Can you work these out from the model? Positions are in its coordinate system, mm. A direction names the side the tool comes from. Give positions to 0.01 mm unless a question says otherwise; leave off trailing zeros. Loops run counter-clockwise (first coordinate to the right, second up) from the corner with the lowest first, then second, coordinate; pieces in that order, holes last. Notation, with made-up numbers: (38.25, 26.25) -> (56.25, 26.25) arc R24 cw to (56.25, 45.25) -> close; hole circle Ø3 at (21, -29). An arc over 180 degrees is marked (long way). Return JSON: item names as keys, results as strings. Group by question number.
Q1. Suppose I cut it at B-B, the plane y = 14.5. Please give me the cut outline in (x, z) (3 decimals), and give its area (3 significant figures).
Q2. Suppose I cut it at C-C, the plane x = 44.5. Please give me the cut outline in (y, z).
Q3. I need wall thicknesses on line 1 along X through (y, z) = (14.75, 5.5) (3 decimals); line 2 along Y through (x, z) = (46.5, 6); line 3 along Z through (x, y) = (28, 4.75). Which ranges of each line are inside material? Lowest first, please. Write a range as [from, to].
Q4. Thinking about a two-plate mould opening in X: for faces 1 (the cylindrical face through (0.285, 1.014, 7.699)), 2 (the cylindrical face through (49.324, 14.986, 7.715)), 3 (the flat face through (2, 15, 8)), which applies, pulls with the +X half, pulls with the -X half, needs draft (parallel to the pull), parting line crosses it, or undercut?
Q5. Will these pins go through, and if not, where does the flat tip stop? pin 1 (8 mm diameter, centred on x = 20.5, y = 3.5, fed in from -Z); pin 2 (1.4 mm diameter, centred on x = 51, y = 1.5, fed in from +Z); pin 3 (8 mm diameter, centred on x = 29.5, y = 11.5, fed in from +Z).
Q6. Which directions (+Z, -Z, +X, -X, +Y, -Y) give clear straight access to the entire face, cutting with the end or side of a thin tool? Please do faces 4 (the flat face through (49, 14, 5)), 5 (the flat face through (50, 1, 2)), 6 (the cylindrical face through (55.215, 15.014, 7.699)).
Q7. Suppose I cut it at A-A, the plane z = 3.75. Count the separate pieces of the cut face and the enclosed holes in it, and give its area (3 significant figures).
```python
from build123d import *

# Parameters (mm, degrees)
BOX001_W     = 1.75
BOX001_H     = 2
BOX001_DEPTH = 10
BOX_W        = 10
BOX_H        = 2
BOX_DEPTH    = 8
FILLET_R     = 1
BOX003_W     = 1.75
BOX003_H     = 2
BOX003_DEPTH = 10
BOX002_W     = 10
BOX002_H     = 2
BOX002_DEPTH = 8
FILLET001_R  = 1
BOX005_W     = 1.75
BOX005_H     = 2
BOX005_DEPTH = 10
BOX004_W     = 10
BOX004_H     = 2
BOX004_DEPTH = 8
FILLET002_R  = 1
BOX007_W     = 1.75
BOX007_H     = 2
BOX007_DEPTH = 10
BOX006_W     = 10
BOX006_H     = 2
BOX006_DEPTH = 8
FILLET003_R  = 1
BOX008_W     = 55.5
BOX008_H     = 16
BOX008_DEPTH = 1.75


with BuildPart() as cube001:
    # Box001 → Box001 (new body)
    with BuildSketch(Plane(origin=(4.125, 0, 2), x_dir=(1, 0, 0), z_dir=(0, 0, 1))):
        with Locations((0.875, 1)):
            Rectangle(BOX001_W, BOX001_H)
    extrude(amount=BOX001_DEPTH)


with BuildPart() as post01:
    # Box → Box (new body)
    with BuildSketch(Plane.XY):
        with Locations((5, 1)):
            Rectangle(BOX_W, BOX_H)
    extrude(amount=BOX_DEPTH)

    # Cut: cut Cube001
    add(cube001.part, mode=Mode.SUBTRACT)

    # Fillet
    fillet_edges = [post01.edges().sort_by_distance(p)[0] for p in [
        (0, 1, 8),
        (4.125, 1, 8),
        (10, 1, 8),
        (5.875, 1, 8),
    ]]
    fillet(fillet_edges, radius=FILLET_R)


with BuildPart() as cube003:
    # Box003 → Box003 (new body)
    with BuildSketch(Plane(origin=(4.125, 0, 2), x_dir=(1, 0, 0), z_dir=(0, 0, 1))):
        with Locations((0.875, 1)):
            Rectangle(BOX003_W, BOX003_H)
    extrude(amount=BOX003_DEPTH)


with BuildPart() as post002:
    # Box002 → Box002 (new body)
    with BuildSketch(Plane.XY):
        with Locations((5, 1)):
            Rectangle(BOX002_W, BOX002_H)
    extrude(amount=BOX002_DEPTH)

    # Cut001: cut Cube003
    add(cube003.part, mode=Mode.SUBTRACT)

    # Fillet001
    fillet001_edges = [post002.edges().sort_by_distance(p)[0] for p in [
        (0, 1, 8),
        (4.125, 1, 8),
        (10, 1, 8),
        (5.875, 1, 8),
    ]]
    fillet(fillet001_edges, radius=FILLET001_R)


with BuildPart() as post002_1:
    # Fillet001 placement: moved
    add(post002.part.moved(Location((0, 14, 0))))


with BuildPart() as cube005:
    # Box005 → Box005 (new body)
    with BuildSketch(Plane(origin=(4.125, 0, 2), x_dir=(1, 0, 0), z_dir=(0, 0, 1))):
        with Locations((0.875, 1)):
            Rectangle(BOX005_W, BOX005_H)
    extrude(amount=BOX005_DEPTH)


with BuildPart() as post003:
    # Box004 → Box004 (new body)
    with BuildSketch(Plane.XY):
        with Locations((5, 1)):
            Rectangle(BOX004_W, BOX004_H)
    extrude(amount=BOX004_DEPTH)

    # Cut002: cut Cube005
    add(cube005.part, mode=Mode.SUBTRACT)

    # Fillet002
    fillet002_edges = [post003.edges().sort_by_distance(p)[0] for p in [
        (0, 1, 8),
        (4.125, 1, 8),
        (10, 1, 8),
        (5.875, 1, 8),
    ]]
    fillet(fillet002_edges, radius=FILLET002_R)


with BuildPart() as post003_1:
    # Fillet002 placement: moved
    add(post003.part.moved(Location((45.5, 0, 0))))


with BuildPart() as cube007:
    # Box007 → Box007 (new body)
    with BuildSketch(Plane(origin=(4.125, 0, 2), x_dir=(1, 0, 0), z_dir=(0, 0, 1))):
        with Locations((0.875, 1)):
            Rectangle(BOX007_W, BOX007_H)
    extrude(amount=BOX007_DEPTH)


with BuildPart() as post004:
    # Box006 → Box006 (new body)
    with BuildSketch(Plane.XY):
        with Locations((5, 1)):
            Rectangle(BOX006_W, BOX006_H)
    extrude(amount=BOX006_DEPTH)

    # Cut003: cut Cube007
    add(cube007.part, mode=Mode.SUBTRACT)

    # Fillet003
    fillet003_edges = [post004.edges().sort_by_distance(p)[0] for p in [
        (0, 1, 8),
        (4.125, 1, 8),
        (10, 1, 8),
        (5.875, 1, 8),
    ]]
    fillet(fillet003_edges, radius=FILLET003_R)


with BuildPart() as post004_1:
    # Fillet003 placement: moved
    add(post004.part.moved(Location((45.5, 14, 0))))


with BuildPart() as axlejig:
    # Box008 → Box008 (new body)
    with BuildSketch(Plane.XY):
        with Locations((27.75, 8)):
            Rectangle(BOX008_W, BOX008_H)
    extrude(amount=BOX008_DEPTH)

    # Fusion: union post01, post002, post003, post004
    add(post01.part)
    add(post002_1.part)
    add(post003_1.part)
    add(post004_1.part)


solid = axlejig.part
```
Ans:
{
 "1": {"outline": "(0, 0) -> (55.5, 0) -> (55.5, 7) arc R1 ccw to (54.5, 8) -> (52.375, 8) arc R1 ccw to (51.375, 7) -> (51.375, 2) -> (49.625, 2) -> (49.625, 7) arc R1 ccw to (48.625, 8) -> (46.5, 8) arc R1 ccw to (45.5, 7) -> (45.5, 1.75) -> (10, 1.75) -> (10, 7) arc R1 ccw to (9, 8) -> (6.875, 8) arc R1 ccw to (5.875, 7) -> (5.875, 2) -> (4.125, 2) -> (4.125, 7) arc R1 ccw to (3.125, 8) -> (1, 8) arc R1 ccw to (0, 7) -> close", "area": "199 mm^2"},
 "2": {"outline": "(0, 0) -> (16, 0) -> (16, 1.75) -> (0, 1.75) -> close"},
 "3": {"line 1": "x = [0, 4.125], [5.875, 10], [45.5, 49.625], [51.375, 55.5]", "line 2": "y = [0, 2], [14, 16]", "line 3": "z = [0, 1.75]"},
 "4": {"face 1": "pulls with the -X half", "face 2": "undercut", "face 3": "needs draft"},
 "5": {"pin 1": "stops at z = 0", "pin 2": "stops at z = 7.74", "pin 3": "stops at z = 1.75"},
 "6": {"face 4": "+Z, +X, -X", "face 5": "+Z, +Y, -Y", "face 6": "+Z, +X, +Y, -Y"},
 "7": {"separate pieces": "8", "enclosed holes": "0", "area": "66.0 mm^2"}
}
